Autodesk Inventor part; units mm, degrees
ref_plane "YZ Plane" through (0, 0, 0) normal (1, 0, 0) x (0, 1, 0)
ref_plane "XZ Plane" through (0, 0, 0) normal (0, 1, 0) x (-1, 0, 0)
ref_plane "XY Plane" through (0, 0, 0) normal (0, 0, 1) x (1, 0, 0)
sketch "スケッチ1" plane through (0, 0, 0) normal (0, 0, 1) x (1, 0, 0)
  circle A0 centre (0, 0) radius 7
  dimension "d0" = 14
extrude "押し出し1" add sketch "スケッチ1" against normal blind 25
sketch "スケッチ2" plane through (0, 0, 0) normal (0, 0, 1) x (1, 0, 0)
  circle A0 centre (0, 0) radius 2
  dimension "d3" = 4
sketch "スケッチ3" plane through (0, 0, -25) normal (0, 0, -1) x (-1, 0, 0)
  circle A0 centre (0, 0) radius 4
  dimension "d4" = 8
extrude "押し出し2" cut sketch "スケッチ3" against normal blind 12.5
extrude "押し出し3" cut sketch "スケッチ2" against normal blind 12.5
fillet "フィレット1" radius 0.5 1 edges at (-7, 0, 0)
fillet "フィレット2" radius 0.5 3 edges at (-2, 0, 0) (-7, 0, -25) (4, 0, -25)
properties part number "4mm-8mmカップリング"
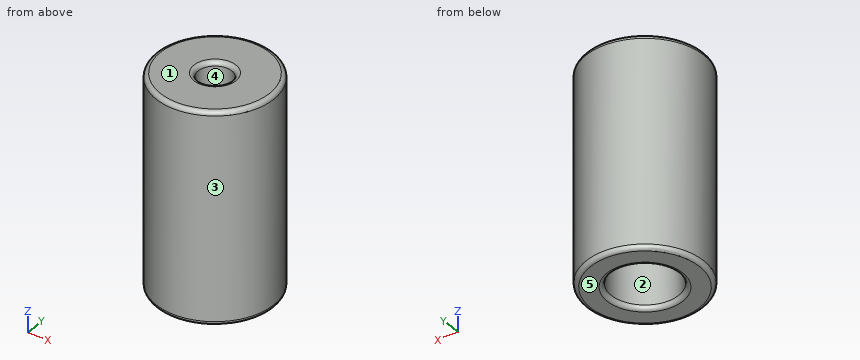
For this review, take the finished solid that the model builds, in its own axes (mm). Face numbers are marked on the shaded views. A direction names the side the tool comes from. Round coordinates to 2 decimals unless told otherwise and drop trailing zeros. Order: outer loops, then holes, each group sorted by start corner. A loop starts at its lowest first (then second) coordinate and runs counter-clockwise, first axis right, second up. Notation, with made-up numbers: (34, 0.25) -> (58, 0.25) arc R17 ccw to (58, 31.25) -> close; hole circle Ø9 at (22.5, -35.5). An arc over 180 degrees is marked (long way). Use a Markdown table: item, result.
Item 1: Take a section at A-A (x = 0). State the section outline as (y, z) points.
Resolved:
| item | result |
|---|---|
| outline | (-7, -24.5) arc R0.5 ccw to (-6.5, -25) -> (-4.5, -25) arc R0.5 ccw to (-4, -24.5) -> (-4, -12.5) -> (-2, -12.5) -> (-2, -0.5) arc R0.5 ccw to (-2.5, 0) -> (-6.5, 0) arc R0.5 ccw to (-7, -0.5) -> close; (2, -12.5) -> (4, -12.5) -> (4, -24.5) arc R0.5 ccw to (4.5, -25) -> (6.5, -25) arc R0.5 ccw to (7, -24.5) -> (7, -0.5) arc R0.5 ccw to (6.5, 0) -> (2.5, 0) arc R0.5 ccw to (2, -0.5) -> close |
Item 2: For pin 1 (1.5 mm diameter, centred on x = -2, z = -20.5, fed in from +Y); pin 2 (2 mm diameter, centred on y = 1.5, z = -20.5, fed in from -X); pin 3 (6.5 mm diameter, centred on x = 0, y = 0, fed in from -Z), all flat-tipped, find the tip position at first contact; note any pin that passes through.
Resolved:
| item | result |
|---|---|
| pin 1 | stops at y = 6.89 |
| pin 2 | stops at x = -6.98 |
| pin 3 | stops at z = -12.5 |
Item 3: Machinability: for the marked faces 1 and 2, which of the approach directions +Z, -Z, +X, -X, +Y, -Y give a long, thin tool a straight path to every point of the face, cutting with its end or side? Answer none if there is none.
Resolved:
| item | result |
|---|---|
| face 1 | +Z, +X, -X, +Y, -Y |
| face 2 | -Z |
Item 4: Take a section at D-D (z = -8.75). State the section outline as (x, y) points.
Resolved:
| item | result |
|---|---|
| outline | circle Ø14 at (0, 0); hole circle Ø4 at (0, 0) |
Item 5: Take a section at C-C (z = -18.5). State the section outline as (x, y) points.
Resolved:
| item | result |
|---|---|
| outline | circle Ø14 at (0, 0); hole circle Ø8 at (0, 0) |
Item 6: Draft analysis for pull direction Y (two halves, no side actions). For the marked faces 3, 4 and 5, state which applies: +Y half, -Y half, draft (parallel to the pull), parting line (faces both ways), or undercut.
Resolved:
| item | result |
|---|---|
| face 3 | parting line |
| face 4 | undercut |
| face 5 | draft |
Item 7: For line 1 along Y through (x, z) = (0, -18); line 2 along Y through (x, z) = (0, -7.75); line 3 along Z through (x, y) = (2.25, 2), list the stretches that pass through material, from the lowest coordinate up. Write a range as [from, to].
Resolved:
| item | result |
|---|---|
| line 1 | y = [-7, -4], [4, 7] |
| line 2 | y = [-7, -2], [2, 7] |
| line 3 | z = [-12.5, 0] |
